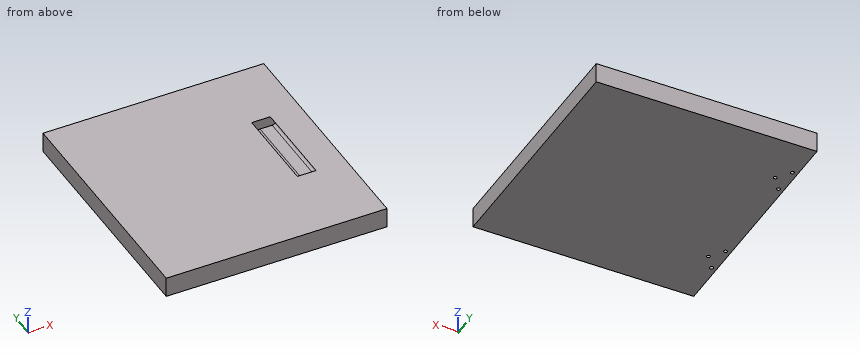
```python
from build123d import *

# Parameters (mm, degrees)
SKETCH1_W               = 325
SKETCH1_H               = 400
BOSS_EXTRUDE1_DEPTH     = 15
SKETCH2_R               = 2.5
CUT_EXTRUDE1_DEPTH      = 10
SKETCH4_W               = 328.47257144
SKETCH4_H               = 49.54
CUT_EXTRUDE3_DEPTH      = 260.434481132
CUT_EXTRUDE4_DEPTH      = 65
MIRROR2_COPY_1_SKETCH_R = 2.5
MIRROR2_COPY_1_DEPTH    = 10
BOSS_EXTRUDE4_REACH     = 261.434
SKETCH6_R               = 2.5


with BuildPart() as part:
    # Sketch1 → Boss-Extrude1 (new, symmetric)
    with BuildSketch(Plane.XY):
        Rectangle(SKETCH1_W, SKETCH1_H)
    extrude(amount=BOSS_EXTRUDE1_DEPTH, both=True)

    # Sketch2 → Cut-Extrude1 (cut)
    with BuildSketch(Plane(origin=(0, 0, -15), x_dir=(-1, 0, 0), z_dir=(0, 0, -1))):
        with Locations((155, 135)):
            Circle(SKETCH2_R)
        with Locations((140, 115)):
            Circle(SKETCH2_R)
        with Locations((155, 95)):
            Circle(SKETCH2_R)
    cut_extrude1 = extrude(amount=-CUT_EXTRUDE1_DEPTH, mode=Mode.SUBTRACT)

    # Mirror1: Cut-Extrude1 across plane
    add(cut_extrude1.mirror(Plane.ZX), mode=Mode.SUBTRACT)

    # Sketch4 → Cut-Extrude3 (cut, through all)
    with BuildSketch(Plane.XY.offset(15)):
        with Locations((1.73628572, 175.23)):
            Rectangle(SKETCH4_W, SKETCH4_H)
    extrude(amount=-CUT_EXTRUDE3_DEPTH, mode=Mode.SUBTRACT)

    # Sketch5 → Cut-Extrude4 (cut, symmetric)
    with BuildSketch(Plane(origin=(0, -19.77, 0), x_dir=(1, 0, 0), z_dir=(0, 1, 0))):
        with BuildLine():
            Line((102.5, 0), (120.5, 0))
            ThreePointArc((120.5, 0), (125.115384615, -3.076923077), (124.050295858, -8.520710059))
            Line((124.050295858, -8.520710059), (111.375739645, -21.301775148))
            ThreePointArc((111.375739645, -21.301775148), (90.961538462, -17.307692308), (102.5, 0))
        make_face()
    extrude(amount=CUT_EXTRUDE4_DEPTH, both=True, mode=Mode.SUBTRACT)

    # Mirror2: Cut-Extrude1 across plane
    add(cut_extrude1.mirror(Plane.ZX.offset(-19.77)), mode=Mode.SUBTRACT)

    # Mirror2 copy 1 sketch → Mirror2 copy 1 (cut)
    with BuildSketch(Plane(origin=(0, -39.54, -15), x_dir=(-1, 0, 0), z_dir=(0, 0, -1))):
        with Locations((155, 135)):
            Circle(MIRROR2_COPY_1_SKETCH_R)
        with Locations((140, 115)):
            Circle(MIRROR2_COPY_1_SKETCH_R)
        with Locations((155, 95)):
            Circle(MIRROR2_COPY_1_SKETCH_R)
    extrude(amount=-MIRROR2_COPY_1_DEPTH, mode=Mode.SUBTRACT)

    # Sketch6 → Boss-Extrude4 (add, up to next)
    with BuildSketch(Plane(origin=(0, 0, -15), x_dir=(-1, 0, 0), z_dir=(0, 0, -1)), mode=Mode.PRIVATE) as boss_extrude4_sk1:
        with Locations((140, 115)):
            Circle(SKETCH6_R)
    boss_extrude4_tool1 = extrude(boss_extrude4_sk1.sketch, amount=-BOSS_EXTRUDE4_REACH, mode=Mode.PRIVATE) - part.part
    # Sketch6 → Boss-Extrude4 (add, up to next)
    with BuildSketch(Plane(origin=(0, 0, -15), x_dir=(-1, 0, 0), z_dir=(0, 0, -1)), mode=Mode.PRIVATE) as boss_extrude4_sk2:
        with Locations((155, 135)):
            Circle(SKETCH6_R)
    boss_extrude4_tool2 = extrude(boss_extrude4_sk2.sketch, amount=-BOSS_EXTRUDE4_REACH, mode=Mode.PRIVATE) - part.part
    # Sketch6 → Boss-Extrude4 (add, up to next)
    with BuildSketch(Plane(origin=(0, 0, -15), x_dir=(-1, 0, 0), z_dir=(0, 0, -1)), mode=Mode.PRIVATE) as boss_extrude4_sk3:
        with Locations((140, -154.54)):
            Circle(SKETCH6_R)
    boss_extrude4_tool3 = extrude(boss_extrude4_sk3.sketch, amount=-BOSS_EXTRUDE4_REACH, mode=Mode.PRIVATE) - part.part
    # Sketch6 → Boss-Extrude4 (add, up to next)
    with BuildSketch(Plane(origin=(0, 0, -15), x_dir=(-1, 0, 0), z_dir=(0, 0, -1)), mode=Mode.PRIVATE) as boss_extrude4_sk4:
        with Locations((155, -174.54)):
            Circle(SKETCH6_R)
    boss_extrude4_tool4 = extrude(boss_extrude4_sk4.sketch, amount=-BOSS_EXTRUDE4_REACH, mode=Mode.PRIVATE) - part.part
    add(boss_extrude4_tool1.solids().sort_by_distance((-140, 115, -15))[0])
    add(boss_extrude4_tool2.solids().sort_by_distance((-155, 135, -15))[0])
    add(boss_extrude4_tool3.solids().sort_by_distance((-140, -154.54, -15))[0])
    add(boss_extrude4_tool4.solids().sort_by_distance((-155, -174.54, -15))[0])


solid = part.part
```
Input: part model. Units: mm. Frame: model coordinates. Round coordinates to 2 decimals unless told otherwise and drop trailing zeros. Loops run counter-clockwise (first coordinate to the right, second up) from the corner with the lowest first, then second, coordinate; pieces in that order, holes last. Notation, with made-up numbers: (-20, 87.5) -> (16, 87.5) arc R24 ccw to (16, 115.5) -> close; hole circle Ø5 at (5.5, -6.5). An arc over 180 degrees is marked (long way). One line per item, written item: value.
(1) Section A-A (y = -52.5). Return the cut outline in (x, z) (3 decimals).
Geometry check:
outline: (-162.5, -15) -> (162.5, -15) -> (162.5, 15) -> (117.625, 15) -> (124.05, 8.521) arc R5 cw to (120.5, 0) -> (102.5, 0) arc R12.5 cw to (90.253, 15) -> (-162.5, 15) -> close
(2) Pin query (flat end, axial travel): pin 1 (4 mm diameter, centred on x = -156, y = -134, fed in from -Z); pin 2 (4 mm diameter, centred on x = -155, y = -95, fed in from -Z). Return the tip coordinate at first contact, or that it passes through.
Geometry check:
pin 1: z = -15
pin 2: z = -5
(3) Material intervals for line 1 (Y direction, x = -155, z = -7.5); line 2 (X direction, y = -115, z = -11.5); line 3 (Z direction, x = 123.5, y = -6), sorted ascending. Write a range as [from, to].
Geometry check:
line 1: [-200, -137.5], [-132.04, -97.5], [-92.5, 52.96], [57.96, 92.5], [97.96, 150.46]
line 2: [-162.5, -142.5], [-137.5, 162.5]
line 3: [-15, 1], [9.08, 15]
